Read the model definition and answer for the solid it produces. Units are mm, in the model's axes. A direction names the side the tool comes from. Give positions to 0.01 mm unless a question says otherwise; leave off trailing zeros. Order: outer loops, then holes, each group sorted by start corner. A loop starts at its lowest first (then second) coordinate and runs counter-clockwise, first axis right, second up. Notation, with made-up numbers: (24, 29) - (82, 29) arc R14 cw to (82, 41) - close; hole circle Ø4 at (28.25, 71). An arc over 180 degrees is marked (long way). Return JSON: item names as keys, results as strings.
```python
from build123d import *

# Parameters (mm, degrees)
BOSS_EXTRUDE1_DEPTH = 10
BOSS_EXTRUDE2_DEPTH = 10


with BuildPart() as part:
    # Sketch1 → Boss-Extrude1 (new body)
    with BuildSketch(Plane.XY):
        with BuildLine():
            Line((-25, 0), (-25, 234.81313371))
            ThreePointArc((-25, 234.81313371), (-17.67766953, 252.49080324), (0, 259.81313371))
            Line((0, 259.81313371), (342.73755676, 259.81313371))
            ThreePointArc((342.73755676, 259.81313371), (360.415226289, 252.49080324), (367.73755676, 234.81313371))
            Line((367.73755676, 234.81313371), (367.73755676, 0))
            ThreePointArc((367.73755676, 0), (360.415226289, -17.67766953), (342.73755676, -25))
            Line((342.73755676, -25), (0, -25))
            ThreePointArc((0, -25), (-17.67766953, -17.67766953), (-25, 0))
        make_face()
        with BuildLine():
            Line((-5, 0), (-5, 156.717467164))
            ThreePointArc((-5, 156.717467164), (8.334411906, 175.574029293), (30.556993535, 169.286474767))
            Line((30.556993535, 169.286474767), (145.055204149, 27.569007604))
            ThreePointArc((145.055204149, 27.569007604), (147.545096107, 6.37967959), (129.498210613, -5))
            Line((129.498210613, -5), (0, -5))
            ThreePointArc((0, -5), (-3.535533906, -3.535533906), (-5, 0))
        make_face(mode=Mode.SUBTRACT)
        with BuildLine():
            Line((66.870567767, 239.81313371), (275.866988993, 239.81313371))
            ThreePointArc((275.866988993, 239.81313371), (293.913874487, 228.43345412), (291.423982529, 207.244126107))
            Line((291.423982529, 207.244126107), (186.925771915, 77.903923741))
            ThreePointArc((186.925771915, 77.903923741), (171.36877838, 70.472931344), (155.811784844, 77.903923741))
            Line((155.811784844, 77.903923741), (51.313574231, 207.244126107))
            ThreePointArc((51.313574231, 207.244126107), (48.823682273, 228.43345412), (66.870567767, 239.81313371))
        make_face(mode=Mode.SUBTRACT)
        with BuildLine():
            Line((347.73755676, 156.717467164), (347.73755676, 0))
            ThreePointArc((347.73755676, 0), (346.273090666, -3.535533906), (342.73755676, -5))
            Line((342.73755676, -5), (213.239346146, -5))
            ThreePointArc((213.239346146, -5), (195.192460652, 6.37967959), (197.682352611, 27.569007604))
            Line((197.682352611, 27.569007604), (312.180563224, 169.286474767))
            ThreePointArc((312.180563224, 169.286474767), (334.403144854, 175.574029293), (347.73755676, 156.717467164))
        make_face(mode=Mode.SUBTRACT)
    extrude(amount=BOSS_EXTRUDE1_DEPTH)

    # Sketch2 → Boss-Extrude2 (add)
    with BuildSketch(Plane.XY.offset(10)):
        with BuildLine():
            Line((342.73755676, 279.81313371), (0, 279.81313371))
            ThreePointArc((0, 279.81313371), (-31.819805153, 266.632938864), (-45, 234.81313371))
            Line((-45, 234.81313371), (-45, 0))
            ThreePointArc((-45, 0), (-31.819805153, -31.819805153), (0, -45))
            Line((0, -45), (342.73755676, -45))
            ThreePointArc((342.73755676, -45), (374.557361913, -31.819805153), (387.73755676, 0))
            Line((387.73755676, 0), (387.73755676, 234.81313371))
            ThreePointArc((387.73755676, 234.81313371), (374.557361913, 266.632938864), (342.73755676, 279.81313371))
        make_face()
        with BuildLine():
            Line((342.73755676, 239.81313371), (0, 239.81313371))
            ThreePointArc((0, 239.81313371), (-3.535533906, 238.348667616), (-5, 234.81313371))
            Line((-5, 234.81313371), (-5, 0))
            ThreePointArc((-5, 0), (-3.535533906, -3.535533906), (0, -5))
            Line((0, -5), (342.73755676, -5))
            ThreePointArc((342.73755676, -5), (346.273090666, -3.535533906), (347.73755676, 0))
            Line((347.73755676, 0), (347.73755676, 234.81313371))
            ThreePointArc((347.73755676, 234.81313371), (346.273090666, 238.348667616), (342.73755676, 239.81313371))
        make_face(mode=Mode.SUBTRACT)
    extrude(amount=BOSS_EXTRUDE2_DEPTH)


solid = part.part
```
Q1. For faces 5 (the cylindrical face through (48.69, 228.15, 4.93)), 6 (the flat face through (169, 259.813, 5)), 7 (the flat face through (174, 239.813, 12)), 8 (the flat face through (367.738, 119, 5)), 9 (the cylindrical face through (360.61, -17.48, 4.93)), determine the directions among +Z, -Z, +X, -X, +Y, -Y from which every point of the face is accessible in a straight line to the end or side of a thin tool.
Values:
{"face 5": "+Z, -Z", "face 6": "-Z, +X, -X, +Y", "face 7": "+Z", "face 8": "-Z, +X, +Y, -Y", "face 9": "-Z, +X, -Y"}
Q2. A cutting plane is placed at D-D (x = 171). Write down the section's boundary in (y, z).
Values:
{"outline": "(-45, 10) - (-25, 10) - (-25, 0) - (70.48, 0) - (70.48, 10) - (-5, 10) - (-5, 20) - (-45, 20) - close; (239.81, 0) - (259.81, 0) - (259.81, 10) - (279.81, 10) - (279.81, 20) - (239.81, 20) - close"}
Q3. A cutting plane is placed at B-B (z = 5.25). Write down the section's boundary in (x, y).
Values:
{"outline": "(-25, 0) arc R25 ccw to (0, -25) - (342.74, -25) arc R25 ccw to (367.74, 0) - (367.74, 234.81) arc R25 ccw to (342.74, 259.81) - (0, 259.81) arc R25 ccw to (-25, 234.81) - close; hole (-5, 0) arc R5 ccw to (0, -5) - (129.5, -5) arc R20 ccw to (145.06, 27.57) - (30.56, 169.29) arc R20 ccw to (-5, 156.72) - close; hole (51.31, 207.24) - (155.81, 77.9) arc R20 ccw to (186.93, 77.9) - (291.42, 207.24) arc R20 ccw to (275.87, 239.81) - (66.87, 239.81) arc R20 ccw to start; hole (197.68, 27.57) arc R20 ccw to (213.24, -5) - (342.74, -5) arc R5 ccw to (347.74, 0) - (347.74, 156.72) arc R20 ccw to (312.18, 169.29) - close"}
Q4. Consider L1, parallel to Y at x = 340.5, z = 17.75; L2, parallel to X at y = 66.5, z = 13.25; L3, parallel to Y at x = 123.5, z = 7.75. Determine where each line is inside the solid, lowest interval first.
Values:
{"L1": "y = -45 to -5, 239.81 to 279.81", "L2": "x = -45 to -5, 347.74 to 387.74", "L3": "y = -25 to -5, 54.25 to 117.9, 239.81 to 259.81"}
Q5. A cutting plane is placed at C-C (y = 189). Write down the section's boundary in (x, z).
Values:
{"outline": "(-45, 10) - (-25, 10) - (-25, 0) - (66.05, 0) - (66.05, 10) - (-5, 10) - (-5, 20) - (-45, 20) - close; (276.68, 0) - (367.74, 0) - (367.74, 10) - (387.74, 10) - (387.74, 20) - (347.74, 20) - (347.74, 10) - (276.68, 10) - close"}
Q6. Determine the mould class of faces 1 (the cylindrical face through (-32.168, -31.468, 14.93)), 2 (the cylindrical face through (374.905, 266.281, 14.93)), 3 (the flat face through (218, 88, 0)), 4 (the flat face through (254.1, 97.4, 4.9)) for opening direction Y: released by +Y, released by -Y, zero draft, split by the parting line, or undercut.
Values:
{"face 1": "released by -Y", "face 2": "released by +Y", "face 3": "zero draft", "face 4": "undercut"}
Q7. A cutting plane is placed at A-A (x = 241). Write down the section's boundary in (y, z).
Values:
{"outline": "(-45, 10) - (-25, 10) - (-25, 0) - (-5, 0) - (-5, 20) - (-45, 20) - close; (81.18, 0) - (144.83, 0) - (144.83, 10) - (81.18, 10) - close; (239.81, 0) - (259.81, 0) - (259.81, 10) - (279.81, 10) - (279.81, 20) - (239.81, 20) - close"}
Q8. Given pin 1 (1.5 mm diameter, centred on y = 232.5, z = 3.5, fed in from -X); pin 2 (3 mm diameter, centred on x = 231.5, z = 7.5, fed in from -Y); pin 3 (1.5 mm diameter, centred on x = 279.5, y = 147.5, fed in from +Z), each flat-ended and moving along its own axis, determine where each tip first touches the part or whether it passes through.
Values:
{"pin 1": "stops at x = -25", "pin 2": "stops at y = -25", "pin 3": "stops at z = 10"}
